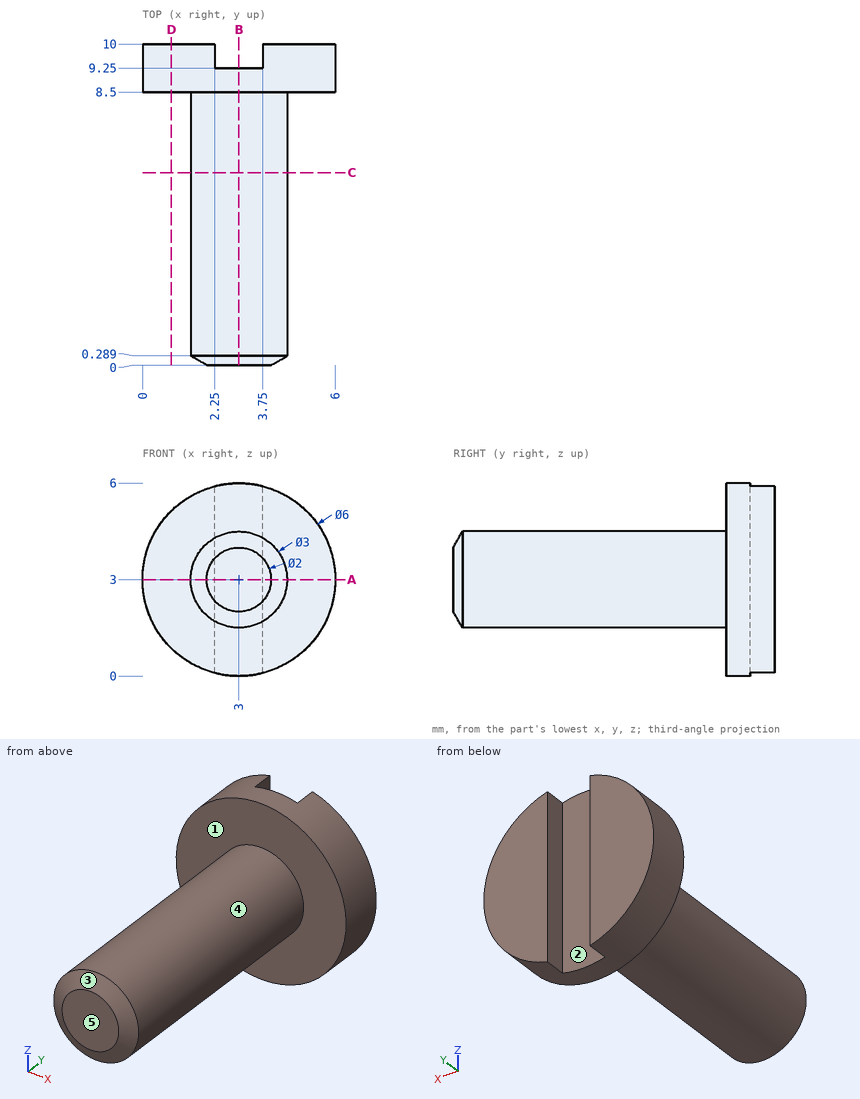
Check sheet for the drawn part. Datum: minimum x, y, z corner. Units: mm. A direction names the side the tool comes from. Give positions to 0.01 mm unless a question says otherwise; leave off trailing zeros. Order: outer loops, then holes, each group sorted by start corner. A loop starts at its lowest first (then second) coordinate and runs counter-clockwise, first axis right, second up. Notation, with made-up numbers: (86, 74.25) -> (128, 74.25) arc R32 ccw to (128, 106.25) -> close; hole circle Ø5 at (62.25, -34). An arc over 180 degrees is marked (long way). Use a Markdown table: item, result.
1) Section check B-B, the plane x = 3. Record the boundary of the cut face in (y, z).
Results:
| item | result |
|---|---|
| outline | (0, 2) -> (0.29, 1.5) -> (8.5, 1.5) -> (8.5, 0) -> (9.25, 0) -> (9.25, 6) -> (8.5, 6) -> (8.5, 4.5) -> (0.29, 4.5) -> (0, 4) -> close |
2) Material ranges on probe 1 along Y at (x, z) = (5.5, 1.4); probe 2 along X at (y, z) = (7.75, 3.1); probe 3 along Z at (x, y) = (1.7, 1.25), recorded low to high.
Results:
| item | result |
|---|---|
| probe 1 | 8.5 to 10 |
| probe 2 | 1.5 to 4.5 |
| probe 3 | 2.25 to 3.75 |
3) Section check C-C, the plane y = 6. Record the boundary of the cut face in (x, z).
Results:
| item | result |
|---|---|
| outline | circle Ø3 at (3, 3) |
4) Depth check by flat-ended pin: pin 1 Ø0.6 at (y, z) = (9.5, 2.5) entering from -X; pin 2 Ø1 at (y, z) = (4, 4.5) entering from +X; pin 3 Ø3 at (y, z) = (6.5, 3.5) entering from -X. Enter the tip coordinate at first touch or a pass-through.
Results:
| item | result |
|---|---|
| pin 1 | x = 0.01 |
| pin 2 | x = 4.12 |
| pin 3 | x = 1.5 |
5) Section check A-A, the plane z = 3. Record the boundary of the cut face in (x, y).
Results:
| item | result |
|---|---|
| outline | (0, 8.5) -> (1.5, 8.5) -> (1.5, 0.29) -> (2, 0) -> (4, 0) -> (4.5, 0.29) -> (4.5, 8.5) -> (6, 8.5) -> (6, 10) -> (3.75, 10) -> (3.75, 9.25) -> (2.25, 9.25) -> (2.25, 10) -> (0, 10) -> close |
6) Mould release check, pull along X, two halves, no side actions. Record for the marked faces 1, 2 and 3: pulls with the +X half, pulls with the -X half, needs draft (parallel to the pull), parting line crosses it, or undercut.
Results:
| item | result |
|---|---|
| face 1 | needs draft |
| face 2 | undercut |
| face 3 | parting line crosses it |
7) Section check D-D, the plane x = 0.9. Record the boundary of the cut face in (y, z).
Results:
| item | result |
|---|---|
| outline | (8.5, 0.86) -> (10, 0.86) -> (10, 5.14) -> (8.5, 5.14) -> close |
8) Tool access check on the marked faces 4 and 5. Record the directions out of +Z, -Z, +X, -X, +Y, -Y that give a thin tool (end or side, any length) a straight path to the whole face; none if there is none.
Results:
| item | result |
|---|---|
| face 4 | -Y |
| face 5 | +Z, -Z, +X, -X, -Y |
